from build123d import *

# Parameters (mm, degrees)
SKETCH1_W                    = 30
SKETCH1_H                    = 57.5
BASE_FLANGE1_DEPTH           = 0.7366
EDGE_FLANGE1_STRIP_CUT_DEPTH = 30
EDGE_FLANGE1_DEPTH           = 30
EDGE_FLANGE2_STRIP_CUT_DEPTH = 79.325030457
EDGE_FLANGE2_DEPTH           = 79.325030457
FILLET1_R                    = 10
CUT_EXTRUDE1_DEPTH           = 126.57552091
CUT_EXTRUDE1_DEPTH_BACK      = 126.57552091
SKETCH14_R                   = 1.984375
CUT_EXTRUDE2_DEPTH           = 126.57552091


# Sheet-metal steps are written as plain solids
with BuildPart() as part:
    # Sketch1 → Base-Flange1 (new body)
    with BuildSketch(Plane(origin=(0, 0, 0), x_dir=(0, 0, -1), z_dir=(1, 0, 0))):
        Rectangle(SKETCH1_W, SKETCH1_H)
    extrude(amount=-BASE_FLANGE1_DEPTH)

    # Edge-Flange1 strip (across the edge) → Edge-Flange1 strip cut (cut)
    with BuildSketch(Plane(origin=(0, 28.75, -15), x_dir=(0.087155742747662, -0.9961946980917452, 0), z_dir=(0, 0, 1))):
        Polygon((-3.794579928, -0.407430966), (0.60820216, -0.792624486), (0.67240108, -0.058827472), (-3.730381008, 0.326366049), align=None)
    extrude(amount=EDGE_FLANGE1_STRIP_CUT_DEPTH, mode=Mode.SUBTRACT)

    # Edge-Flange1 section (across the edge) → Edge-Flange1 (add)
    with BuildSketch(Plane(origin=(0, 28.75, -15), x_dir=(0.087155742747662, -0.9961946980917452, 0), z_dir=(0, 0, 1))):
        with BuildLine():
            Line((-0.7366, 0.674969543), (-0.7366, 80))
            Line((-0.7366, 80), (0, 80))
            Line((0, 80), (0, 0.674969543))
            ThreePointArc((0, 0.674969543), (0.193521514, 0.177329796), (0.67240108, -0.058827472))
            Line((0.67240108, -0.058827472), (0.60820216, -0.792624486))
            ThreePointArc((0.60820216, -0.792624486), (-0.349556973, -0.320309951), (-0.7366, 0.674969543))
        make_face()
    extrude(amount=EDGE_FLANGE1_DEPTH)

    # Edge-Flange2 strip (across the edge) → Edge-Flange2 strip cut (cut)
    with BuildSketch(Plane(origin=(0.60820216, 29.542624486, 15), x_dir=(-0.015134435901339633, 0.17298739392509335, -0.9848077530122075), z_dir=(0.9961946980917453, 0.08715574274766204, 0))):
        Polygon((-3.871674841, -0.065282507), (0.480781505, -0.832737993), (0.608690752, -0.107328603), (-3.743765593, 0.660126883), align=None)
    edge_flange2_strip_cut = extrude(amount=EDGE_FLANGE2_STRIP_CUT_DEPTH, mode=Mode.SUBTRACT)

    # Edge-Flange2 section (across the edge) → Edge-Flange2 (add)
    with BuildSketch(Plane(origin=(0.60820216, 29.542624486, 15), x_dir=(-0.015134435901339633, 0.17298739392509335, -0.9848077530122075), z_dir=(0.9961946980917453, 0.08715574274766204, 0))):
        with BuildLine():
            Line((-0.7366, 0.618080788), (-0.7366, 59))
            Line((-0.7366, 59), (0, 59))
            Line((0, 59), (0, 0.618080788))
            ThreePointArc((0, 0.618080788), (0.172331663, 0.144603435), (0.608690752, -0.107328603))
            Line((0.608690752, -0.107328603), (0.480781505, -0.832737993))
            ThreePointArc((0.480781505, -0.832737993), (-0.391936674, -0.328873918), (-0.7366, 0.618080788))
        make_face()
    edge_flange2 = extrude(amount=EDGE_FLANGE2_DEPTH)

    # Mirror1: Edge-Flange2 strip cut, Edge-Flange2 across plane
    add(edge_flange2_strip_cut.mirror(Plane.XY), mode=Mode.SUBTRACT)
    add(edge_flange2.mirror(Plane.XY))

    # Fillet1
    fillet1_edges = [part.edges().sort_by_distance(p)[0] for p in [
        (74.572883521, 94.275100646, -25.607947178),
        (-4.450291247, 87.361468698, -25.607947178),
        (-4.450291247, 87.361468698, 25.607947178),
        (74.572883521, 94.275100646, 25.607947178),
    ]]
    fillet(fillet1_edges, radius=FILLET1_R)

    # Sketch13 → Cut-Extrude1 (cut, two sides: drawn at the far end of the back side and taken through both)
    with BuildSketch(Plane(origin=(0, 0, 0), x_dir=(0, 0, -1), z_dir=(1, 0, 0)).offset(-CUT_EXTRUDE1_DEPTH_BACK)):
        Polygon((276.166836222, -21.75), (15, -21.75), (7, -21.75), (-2.746794345, -28.75), (-214.875081206, -181.097321129), (-53.649855395, -677.926156777), (437.392062033, -518.578835647), align=None)
    extrude(amount=CUT_EXTRUDE1_DEPTH + CUT_EXTRUDE1_DEPTH_BACK, mode=Mode.SUBTRACT)

    # Sketch14 → Cut-Extrude2 (cut, through all)
    with BuildSketch(Plane(origin=(0, 0, 0), x_dir=(0, 0, -1), z_dir=(1, 0, 0))):
        with Locations((-7.5, -10.75)):
            Circle(SKETCH14_R)
        with Locations((7.5, -10.75)):
            Circle(SKETCH14_R)
    extrude(amount=-CUT_EXTRUDE2_DEPTH, mode=Mode.SUBTRACT)


solid = part.part
Build history of the part. All positions in model axes, mm. A direction names the side the tool comes from. Round coordinates to 2 decimals unless told otherwise and drop trailing zeros. Loops run counter-clockwise (first coordinate to the right, second up) from the corner with the lowest first, then second, coordinate; pieces in that order, holes last. Notation, with made-up numbers: (86, 42) -> (98, 42) arc R23 ccw to (98, 66) -> close; hole circle Ø10 at (20.5, 53). An arc over 180 degrees is marked (long way). One line per item, written item: value. Start each with the question number.
Q1. 3-axis set-ups, long thin cutter, end or side, ignore diameter. For faces 1 (the face through (-0.363, -12.687, -7.07)), 2 (the face through (39.551, 33.127, 14.861)): which of +Z, -Z, +X, -X, +Y, -Y reach the whole face in a straight line?
Q2. Cut at D-D on z = 1. List the corners of the cut face in (x, y).
Q3. Probe line 1 along Y through (x, z) = (-0.55, -7.5); line 2 along Y through (x, z) = (-0.5, -7.5); line 3 along Z through (x, y) = (64, 85.5). List the from-to ranges inside material, lowest first.
Q4. Cut at B-B on z = 7.5. List the corners of the cut face in (x, y), plus the area to 3 significant figures.
Q5. Cut at A-A on y = -10.75. List the corners of the cut face in (x, z), plus the area to 3 significant figures.
Q6. Two-plate mould, pull along Y, no slides. Class faces 3 (the face through (39.602, 32.551, -15.318)), 4 (the face through (71.99, 91.08, 25.08)), 5 (the face through (-0.36, -12.51, 6.58)): released by +Y, released by -Y, zero draft, split by the parting line, or undercut.
Q7. Cut at C-C on y = 49. List the corners of the cut face in (x, z).
Q8. Drop flat-ended pins along their axis: pin 1 Ø1 at (x, z) = (27, 6.5) entering from +Y; pin 2 Ø12 at (y, z) = (34.5, -8.5) entering from -X; pin 3 Ø3 at (y, z) = (-10.75, -7.5) entering from -X; pin 4 Ø10 at (x, z) = (50, -6.5) entering from -Y. Give the stop position or say it passes through.
Computed:
1. face 1: +X, -X
1. face 2: -X, +Y
2. outline: (-0.74, -27.5) -> (0, -27.5) -> (0, 28.08) arc R0.74 cw to (0.67, 28.81) -> (79.7, 35.72) -> (79.63, 36.46) -> (0.61, 29.54) arc R1.47 ccw to (-0.74, 28.08) -> close
3. line 1: -21.75 to -12.73, -8.77 to 28.79
3. line 2: -21.75 to -12.73, -8.77 to 28.88
3. line 3: -24.6 to -23.86, 23.86 to 24.6
4. outline: (-0.74, -28.75) -> (0, -28.75) -> (0, -12.73) -> (-0.74, -12.73) -> close; (-0.74, -8.77) -> (0, -8.77) -> (0, 28.08) arc R0.74 cw to (0.67, 28.81) -> (79.7, 35.72) -> (79.63, 36.46) -> (0.61, 29.54) arc R1.47 ccw to (-0.74, 28.08) -> close
4. area: 98.6 mm²
5. outline: (-0.74, -15) -> (0, -15) -> (0, -9.48) -> (-0.74, -9.48) -> close; (-0.74, -5.52) -> (0, -5.52) -> (0, 5.52) -> (-0.74, 5.52) -> close; (-0.74, 9.48) -> (0, 9.48) -> (0, 15) -> (-0.74, 15) -> close
5. area: 16.3 mm²
6. face 3: released by -Y
6. face 4: released by +Y
6. face 5: undercut
7. outline: (-1.09, -19.19) -> (78.53, -17.97) -> (78.53, -17.22) -> (-1.09, -18.44) -> close; (-1.09, 18.44) -> (78.53, 17.22) -> (78.53, 17.97) -> (-1.09, 19.19) -> close
8. pin 1: y = 31.9
8. pin 2: x = -0.67
8. pin 3: through
8. pin 4: y = 32.69
